Part model, mm, in its own coordinate system. A direction names the side the tool comes from. Give positions to 0.01 mm unless a question says otherwise; leave off trailing zeros. Write each loop counter-clockwise with the first axis right and the second up, starting at its lowest first coordinate (ties: lowest second). Pieces come first, ordered by that corner, then holes. Notation, with made-up numbers: M -27,46 L 9,46 A34 ccw 9,84 Z; hole C -35.5,14.25 d11. An arc over 180 degrees is marked long. Use CSV: the item, a comma, the result in double quotes. Start each with the question number.
Item 1: Cut at B-B (z = 37). List the corners of the cut face in (x, y), then the cut area to 3 significant figures.
Item 2: Cut at A-A (x = -2). List the corners of the cut face in (y, z).
Item 3: Pin check, flat tips, straight feed: pin 1 (6 mm diameter, centred on x = 5, y = 16, fed in from +Z); pin 2 (3 mm diameter, centred on x = -1, y = 36.5, fed in from -Z); pin 3 (6 mm diameter, centred on x = 1, y = 23.5, fed in from +Z). Stop position of each tip, or through.
Item 4: Drill centre lines: line 1 (Y direction, x = -0.5, z = -144); line 2 (X direction, y = -48, z = 95); line 3 (Z direction, x = -8.75, y = 29.5). Where is each one in solid material? Low to high. Write a range as [from, to].
Item 5: Which spindle directions (+Z, -Z, +X, -X, +Y, -Y) get a long thin tool onto all of the face, cutting with end or side? Do faces 1 (the flat face through (0, 53, -210.125)), 2 (the cylindrical face through (-2.17, 9.76, -0.91)), 3 (the cylindrical face through (-2.168, -42.912, 158.994)), 4 (the cylindrical face through (-2.168, 62.436, -160.405)). Say none if no direction does.
from build123d import *

# Parameters (mm, degrees)
SKETCH3_R = 10


with BuildPart() as part:
    # Sweep2: sweep along a path in Sketch1
    with BuildLine(Plane(origin=(0, 0, 0), x_dir=(0, 0, -1), z_dir=(1, 0, 0))) as sweep2_path:
        Line((-210.124764734, -52.674246303), (-160.124764734, -52.674246303))
        Line((-160.124764734, -52.674246303), (-109.274248541, -52.674246303))
        ThreePointArc((-109.274248541, -52.674246303), (-91.582896902, -44.460377319), (-86.440777952, -25.64521909))
        ThreePointArc((-86.440777952, -25.64521909), (-81.561920639, -7.793342617), (-64.776315105, 0))
        Line((-64.776315105, 0), (64.776315105, 0))
        ThreePointArc((64.776315105, 0), (81.561920639, 7.793342617), (86.440777952, 25.64521909))
        ThreePointArc((86.440777952, 25.64521909), (91.582896902, 44.460377319), (109.274248541, 52.674246303))
        Line((109.274248541, 52.674246303), (160.124764734, 52.674246303))
        Line((160.124764734, 52.674246303), (210.124764734, 52.674246303))
    # Sketch3 → Sweep2 (sweep)
    with BuildSketch(Plane(origin=(0, -52.674246303, 210.124764734), x_dir=(1, 0, 0), z_dir=(0, 0, 1))):
        Circle(SKETCH3_R)
    sweep(path=sweep2_path.line)


solid = part.part
Worked answers:
1,outline,"C 0,0 d20"
1,area,"314 mm^2"
2,outline,"M -62.47,109.27 A32.96 ccw -24.01,76.78 A12.18 cw -9.8,64.78 L -9.8,-64.78 A31.77 ccw 27.28,-96.1 A13.36 cw 42.88,-109.27 L 42.88,-210.12 L 62.47,-210.12 L 62.47,-109.27 A32.96 ccw 24.01,-76.78 A12.18 cw 9.8,-64.78 L 9.8,64.78 A31.77 ccw -27.28,96.1 A13.36 cw -42.88,109.27 L -42.88,210.12 L -62.47,210.12 Z"
3,pin 1,"stops at z = -74.02"
3,pin 2,"stops at z = -99.16"
3,pin 3,"stops at z = -76.26"
4,line 1,"y = [42.69, 62.66]"
4,line 2,"x = [-10, 10]"
4,line 3,"z = [-90.96, -81.27]"
5,face 1,"-Z, +X, -X, +Y, -Y"
5,face 2,"none"
5,face 3,"+Z"
5,face 4,"-Z"
